Geometry check sheet. Reference: the model listing, model coordinates, mm. A direction names the side the tool comes from. Round coordinates to 2 decimals unless told otherwise and drop trailing zeros. Loops run counter-clockwise (first coordinate to the right, second up) from the corner with the lowest first, then second, coordinate; pieces in that order, holes last. Notation, with made-up numbers: M -37.5,-15.5 L -10.5,-15.5 A12 cw -10.5,-10.5 Z; hole C 16,9 d3. An arc over 180 degrees is marked long. Answer in a Markdown table with one row per item. Add a question column.
```python
from build123d import *

# Parameters (mm, degrees)
BASPROSKE_W             = 6
BASPROSKE_H             = 16.5
TOOTHCUT_DEPTH          = 25.093567606
TEETHCUTS_COUNT         = 20
TEETHCUTS_ANGLE         = 342
BORSKE_R                = 3.1
BORE_DEPTH              = 50.0000508
BOSS_EXTRU_1_DEPTH      = 6
ESQUISSE3_R             = 0.75
ENL_V_MAT_EXTRU_1_DEPTH = 6


with BuildPart() as part:
    # BasProSke → Base-Revolve (revolve)
    with BuildSketch(Plane(origin=(0, 0, 0), x_dir=(1, 0, 0), z_dir=(0, 1, 0)), mode=Mode.PRIVATE) as base_revolve_sk:
        with Locations((3, 8.25)):
            Rectangle(BASPROSKE_W, BASPROSKE_H)
    revolve(base_revolve_sk.sketch.rotate(Axis((-10, 0, 0), (1, 0, 0)), 180), axis=Axis((-10, 0, 0), (1, 0, 0)))

    # TooCutSke → ToothCut (cut, through all)
    with BuildSketch(Plane(origin=(0, 0, 0), x_dir=(0, 0, -1), z_dir=(1, 0, 0))):
        with BuildLine():
            ThreePointArc((0.74381438, 13.102904875), (0, 13.124), (-0.74381438, 13.102904875))
            ThreePointArc((-0.74381438, 13.102904875), (-1.226473103, 14.852072512), (-2.209965745, 16.376962373))
            ThreePointArc((-2.209965745, 16.376962373), (0, 16.5254), (2.209965745, 16.376962373))
            ThreePointArc((2.209965745, 16.376962373), (1.226473103, 14.852072512), (0.74381438, 13.102904875))
        make_face()
    toothcut = extrude(amount=TOOTHCUT_DEPTH, mode=Mode.SUBTRACT)

    # TeethCuts: ToothCut ×20 about axis, 6 skipped
    teethcuts_axis = Axis((-10, 0, 0), (1, 0, 0))
    add([toothcut.rotate(teethcuts_axis, i * TEETHCUTS_ANGLE / (TEETHCUTS_COUNT - 1)) for i in range(1, TEETHCUTS_COUNT) if i not in (12, 13, 14, 15, 16, 17)], mode=Mode.SUBTRACT)

    # BorSke → Bore (cut, symmetric)
    with BuildSketch(Plane(origin=(0, 0, 0), x_dir=(0, 0, -1), z_dir=(1, 0, 0))):
        with Locations(Location((0, 0, 0), (0, 0, 180))):
            Circle(BORSKE_R)
    extrude(amount=BORE_DEPTH, both=True, mode=Mode.SUBTRACT)

    # Esquisse2 → Boss.-Extru.1 (add)
    with BuildSketch(Plane(origin=(6, 0, 0), x_dir=(0, 0, -1), z_dir=(1, 0, 0))):
        Polygon((10.44563255, 6.017449598), (8.099115574, -8.797875511), (44.238631957, -14.521812587), (46.585148932, 0.293512522), align=None)
    extrude(amount=-BOSS_EXTRU_1_DEPTH)

    # Esquisse3 → Enlèv. mat.-Extru.1 (cut)
    with BuildSketch(Plane.ZY):
        with Locations((8, 0)):
            Circle(ESQUISSE3_R)
        with Locations((-8, 0)):
            Circle(ESQUISSE3_R)
        with Locations((0, 8)):
            Circle(ESQUISSE3_R)
        with Locations((0, -8)):
            Circle(ESQUISSE3_R)
    extrude(amount=-ENL_V_MAT_EXTRU_1_DEPTH, mode=Mode.SUBTRACT)


solid = part.part
```
1) Go/stop test with flat-tipped pins: pin 1 (1.2 mm diameter, centred on y = -8, z = 0, fed in from -X); pin 2 (1.5 mm diameter, centred on x = 2.5, z = 0.5, fed in from +Y). Record where each tip stops, or that it passes through.
2) Cross-section at C-C, the plane z = -12.5. Record the boundary of the cut face in (x, y).
3) Set-up check for faces 4 (the cylindrical face through (2.958, -1.21, 14.815)), 5 (the cylindrical face through (2.958, -14.514, -3.422)), 6 (the cylindrical face through (2.958, 11.274, 9.687)), 7 (the flat face through (3.042, -12.045, -28.6)): record each of +Z, -Z, +X, -X, +Y, -Y from which the full face is reachable in a straight line by a thin tool's end or side.
4) Cross-section at D-D, the plane y = 6.5. Record the boundary of the cut face in (x, z).
5) Cross-section at B-B, the plane x = 2.05. Count the separate pieces of the cut face and the enclosed holes in it, plus the area to 3 significant figures.
6) Draft check along Y on faces 1 (the cylindrical face through (2.958, -14.464, 3.427)), 2 (the cylindrical face through (2.958, -14.815, -1.21)), 3 (the cylindrical face through (3, 14, -6)). Enter one of: +Y half, -Y half, draft (parallel to the pull), parting line (faces both ways), or undercut.
7) Thickness scan on L1, parallel to Y at x = 2.2, z = 0; L2, parallel to Y at x = 2.65, z = -8; L3, parallel to Y at x = 4.7, z = 8. Record the ranges inside material, lowest first. Write a range as [from, to].
8) Cross-section at A-A, the plane z = 0. Record the boundary of the cut face in (x, y).
Worked answers:
| question | item | result |
|---|---|---|
| 1 | pin 1 | passes through |
| 1 | pin 2 | stops at y = 14.9 |
| 2 | outline | M 0,-10.77 L 6,-10.77 L 6,10.77 L 0,10.77 Z |
| 3 | face 4 | +Z, +X, -X |
| 3 | face 5 | +X, -X |
| 3 | face 6 | +X, -X, +Y |
| 3 | face 7 | +X, -X, -Y |
| 4 | outline | M 0,-15.17 L 6,-15.17 L 6,14.44 L 0,14.44 Z |
| 5 | separate pieces | 1 |
| 5 | enclosed holes | 5 |
| 5 | area | 1,150 mm2 |
| 6 | face 1 | undercut |
| 6 | face 2 | -Y half |
| 6 | face 3 | +Y half |
| 7 | L1 | y = [-13.12, -8.75], [-7.25, -3.1], [3.1, 7.25], [8.75, 13.12] |
| 7 | L2 | y = [-14.43, -0.75], [0.75, 10.4] |
| 7 | L3 | y = [-10.4, -0.75], [0.75, 10.4] |
| 8 | outline | M 0,-13.12 L 6,-13.12 L 6,-8.75 L 0,-8.75 Z; M 0,-7.25 L 6,-7.25 L 6,-3.1 L 0,-3.1 Z; M 0,3.1 L 6,3.1 L 6,7.25 L 0,7.25 Z; M 0,8.75 L 6,8.75 L 6,13.12 L 0,13.12 Z |
